Check sheet for the modelled part. Datum: model origin and axes. Units: mm. Round coordinates to 2 decimals unless told otherwise and drop trailing zeros. Write each loop counter-clockwise with the first axis right and the second up, starting at its lowest first coordinate (ties: lowest second). Pieces come first, ordered by that corner, then holes. Notation, with made-up numbers: (82.5, 76) - (102.5, 76) arc R35 ccw to (102.5, 111) - close; hole circle Ø1 at (15.25, -2.75). An arc over 180 degrees is marked (long way). Use one line per item in the form item = value. Start each with the question number.
1) Section check C-C (z = -50). Record the boundary of the cut face in (x, y).
2) Section check B-B (z = -68.5). Record the boundary of the cut face in (x, y), then the cut area to 3 significant figures.
3) Scan lines: probe 1 along X at (y, z) = (1.6, -70); probe 2 along Z at (x, y) = (9, 3.55); probe 3 along X at (y, z) = (2.6, -53.2). Record each from-to range of solid material in increasing order.
4) Section check D-D (x = 49). Record the boundary of the cut face in (y, z).
5) Gauge pin test, flat ends, axial feed: P1, Ø1, axis at y = 2, z = -18, coming from the +X side; P2, Ø2.5, axis at y = 2, z = -86, coming from the -X side. Record the tip position at first contact, or that the pin passes through.
6) Section check A-A (x = 101). Record the boundary of the cut face in (y, z).
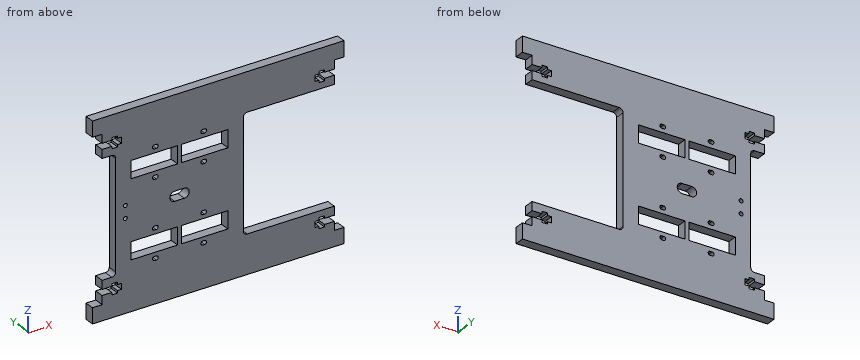
from build123d import *

# Parameters (mm, degrees)
SKETCH1_W           = 120
SKETCH1_H           = 100
SKETCH1_W_2         = 50
SKETCH1_H_2         = 9
BOSS_EXTRUDE1_DEPTH = 5
SKETCH2_W           = 5
SKETCH2_H           = 8
BOSS_EXTRUDE2_DEPTH = 5
SKETCH3_W           = 47
SKETCH3_H           = 60
SKETCH3_W_2         = 7
CUT_EXTRUDE1_DEPTH  = 161.15617378
FILLET1_R           = 2
SKETCH4_R           = 1
CUT_EXTRUDE2_DEPTH  = 161.15617378
CUT_EXTRUDE3_DEPTH  = 161.15617378
SKETCH6_W           = 2
SKETCH6_H           = 9
BOSS_EXTRUDE3_DEPTH = 5


with BuildPart() as part:
    # Sketch1 → Boss-Extrude1 (new body)
    with BuildSketch(Plane(origin=(0, 0, 0), x_dir=(1, 0, 0), z_dir=(0, 1, 0))):
        with Locations((60, 50)):
            Rectangle(SKETCH1_W, SKETCH1_H)
        with BuildLine():
            Line((27, 78.5), (28, 78.5))
            ThreePointArc((28, 78.5), (29, 77.5), (28, 76.5))
            Line((28, 76.5), (27, 76.5))
            ThreePointArc((27, 76.5), (26, 77.5), (27, 78.5))
        make_face(mode=Mode.SUBTRACT)
        with Locations((40, 70)):
            Rectangle(SKETCH1_W_2, SKETCH1_H_2, mode=Mode.SUBTRACT)
        with BuildLine():
            Line((53, 78.5), (52, 78.5))
            ThreePointArc((52, 78.5), (51, 77.5), (52, 76.5))
            Line((52, 76.5), (53, 76.5))
            ThreePointArc((53, 76.5), (54, 77.5), (53, 78.5))
        make_face(mode=Mode.SUBTRACT)
        with BuildLine():
            Line((27, 61.5), (28, 61.5))
            ThreePointArc((28, 61.5), (29, 62.5), (28, 63.5))
            Line((28, 63.5), (27, 63.5))
            ThreePointArc((27, 63.5), (26, 62.5), (27, 61.5))
        make_face(mode=Mode.SUBTRACT)
        with BuildLine():
            Line((53, 61.5), (52, 61.5))
            ThreePointArc((52, 61.5), (51, 62.5), (52, 63.5))
            Line((52, 63.5), (53, 63.5))
            ThreePointArc((53, 63.5), (54, 62.5), (53, 61.5))
        make_face(mode=Mode.SUBTRACT)
        with BuildLine():
            Line((27, 21.5), (28, 21.5))
            ThreePointArc((28, 21.5), (29, 22.5), (28, 23.5))
            Line((28, 23.5), (27, 23.5))
            ThreePointArc((27, 23.5), (26, 22.5), (27, 21.5))
        make_face(mode=Mode.SUBTRACT)
        with BuildLine():
            Line((53, 21.5), (52, 21.5))
            ThreePointArc((52, 21.5), (51, 22.5), (52, 23.5))
            Line((52, 23.5), (53, 23.5))
            ThreePointArc((53, 23.5), (54, 22.5), (53, 21.5))
        make_face(mode=Mode.SUBTRACT)
        with BuildLine():
            Line((27, 38.5), (28, 38.5))
            ThreePointArc((28, 38.5), (29, 37.5), (28, 36.5))
            Line((28, 36.5), (27, 36.5))
            ThreePointArc((27, 36.5), (26, 37.5), (27, 38.5))
        make_face(mode=Mode.SUBTRACT)
        with BuildLine():
            Line((53, 38.5), (52, 38.5))
            ThreePointArc((52, 38.5), (51, 37.5), (52, 36.5))
            Line((52, 36.5), (53, 36.5))
            ThreePointArc((53, 36.5), (54, 37.5), (53, 38.5))
        make_face(mode=Mode.SUBTRACT)
        with Locations((40, 30)):
            Rectangle(SKETCH1_W_2, SKETCH1_H_2, mode=Mode.SUBTRACT)
    extrude(amount=BOSS_EXTRUDE1_DEPTH)

    # Sketch2 → Boss-Extrude2 (add)
    with BuildSketch(Plane(origin=(0, 5, 0), x_dir=(1, 0, 0), z_dir=(0, 1, 0))):
        with Locations((122.5, 96)):
            Rectangle(SKETCH2_W, SKETCH2_H)
        with Locations((122.5, 4)):
            Rectangle(SKETCH2_W, SKETCH2_H)
        with Locations((-2.5, 4)):
            Rectangle(SKETCH2_W, SKETCH2_H)
        with Locations((-2.5, 96)):
            Rectangle(SKETCH2_W, SKETCH2_H)
    extrude(amount=-BOSS_EXTRUDE2_DEPTH)

    # Sketch3 → Cut-Extrude1 (cut, through all)
    with BuildSketch(Plane(origin=(0, 5, 0), x_dir=(1, 0, 0), z_dir=(0, 1, 0))):
        with Locations((96.5, 50)):
            Rectangle(SKETCH3_W, SKETCH3_H)
        with Locations((3.5, 50)):
            Rectangle(SKETCH3_W_2, SKETCH3_H)
    extrude(amount=-CUT_EXTRUDE1_DEPTH, mode=Mode.SUBTRACT)

    # Fillet1
    fillet1_edges = [part.edges().sort_by_distance(p)[0] for p in [
        (73, 2.5, -20),
        (73, 2.5, -80),
        (7, 2.5, -80),
        (7, 2.5, -20),
    ]]
    fillet(fillet1_edges, radius=FILLET1_R)

    # Sketch4 → Cut-Extrude2 (cut, through all)
    with BuildSketch(Plane(origin=(0, 5, 0), x_dir=(1, 0, 0), z_dir=(0, 1, 0))):
        with Locations(Location((12, 53.2, 0), (0, 0, 270))):
            Circle(SKETCH4_R)
        with Locations(Location((12, 46.8, 0), (0, 0, 270))):
            Circle(SKETCH4_R)
        with BuildLine():
            Line((37.5, 52.5), (42.5, 52.5))
            ThreePointArc((42.5, 52.5), (45, 50), (42.5, 47.5))
            Line((42.5, 47.5), (37.5, 47.5))
            ThreePointArc((37.5, 47.5), (35, 50), (37.5, 52.5))
        make_face()
    extrude(amount=-CUT_EXTRUDE2_DEPTH, mode=Mode.SUBTRACT)

    # Sketch5 → Cut-Extrude3 (cut, through all)
    with BuildSketch(Plane(origin=(0, 5, 0), x_dir=(1, 0, 0), z_dir=(0, 1, 0))):
        Polygon((120, 15.5), (115, 15.5), (115, 16.75), (112, 16.75), (112, 15.5), (110, 15.5), (110, 12.5), (112, 12.5), (112, 11.25), (115, 11.25), (115, 12.5), (120, 12.5), align=None)
        Polygon((0, 12.5), (0, 15.5), (5, 15.5), (5, 16.75), (8, 16.75), (8, 15.5), (10, 15.5), (10, 12.5), (8, 12.5), (8, 11.25), (5, 11.25), (5, 12.5), align=None)
        Polygon((0, 84.5), (5, 84.5), (5, 83.25), (8, 83.25), (8, 84.5), (10, 84.5), (10, 87.5), (8, 87.5), (8, 88.75), (5, 88.75), (5, 87.5), (0, 87.5), align=None)
        Polygon((120, 87.5), (120, 84.5), (115, 84.5), (115, 83.25), (112, 83.25), (112, 84.5), (110, 84.5), (110, 87.5), (112, 87.5), (112, 88.75), (115, 88.75), (115, 87.5), align=None)
    extrude(amount=-CUT_EXTRUDE3_DEPTH, mode=Mode.SUBTRACT)

    # Sketch6 → Boss-Extrude3 (add)
    with BuildSketch(Plane(origin=(0, 5, 0), x_dir=(1, 0, 0), z_dir=(0, 1, 0))):
        with Locations((40, 70)):
            Rectangle(SKETCH6_W, SKETCH6_H)
        with Locations((40, 30)):
            Rectangle(SKETCH6_W, SKETCH6_H)
    extrude(amount=-BOSS_EXTRUDE3_DEPTH)


solid = part.part
Results are:
q1.outline = (7, 0) - (35, 0) - (35, 5) - (7, 5) - close; (45, 0) - (73, 0) - (73, 5) - (45, 5) - close
q2.outline = (7, 0) - (15, 0) - (15, 5) - (7, 5) - close; (39, 0) - (41, 0) - (41, 5) - (39, 5) - close; (65, 0) - (73, 0) - (73, 5) - (65, 5) - close
q2.area = 90.0 mm²
q3.probe_1 = 7 to 15, 39 to 41, 65 to 73
q3.probe_2 = -100 to -87.5, -84.5 to -15.5, -12.5 to 0
q3.probe_3 = 7 to 11, 13 to 73
q4.outline = (0, -100) - (5, -100) - (5, -74.5) - (0, -74.5) - close; (0, -65.5) - (5, -65.5) - (5, -34.5) - (0, -34.5) - close; (0, -25.5) - (5, -25.5) - (5, 0) - (0, 0) - close
q5.P1 = 120
q5.P2 = 10
q6.outline = (0, -100) - (5, -100) - (5, -80) - (0, -80) - close; (0, -20) - (5, -20) - (5, 0) - (0, 0) - close
